Part model, mm, in its own coordinate system. A direction names the side the tool comes from. Round coordinates to 2 decimals unless told otherwise and drop trailing zeros. Loops run counter-clockwise (first coordinate to the right, second up) from the corner with the lowest first, then second, coordinate; pieces in that order, holes last.
1) Band-saw the part on C-C, the plane z = 8.25. Write the cut outline in (x, y).
2) 3-axis set-ups, long thin cutter, end or side, ignore diameter. For faces 1 (the flat face through (0, 8, 5)), 2 (the cylindrical face through (0, 2, 12)): which of +Z, -Z, +X, -X, +Y, -Y reach the whole face in a straight line?
3) Mould opens along Z. For faces 3 (the conical face through (-0.1, -5.2, 0.2)), 4 (the flat face through (0, 8, 13)), 5 (the flat face through (0, 3, 21)) say: +Z half, -Z half, draft (parallel to the pull), parting line (faces both ways), or undercut.
4) Band-saw the part on B-B, the plane z = 4.25. Write the cut outline in (x, y), then the cut area to 3 significant figures.
5) Probe line 1 (Z direction, x = 3, y = 7.5); line 2 (Y direction, x = 0, z = 8.5); line 3 (Y direction, x = 0, z = 15). List the from-to ranges inside material, lowest first.
6) Drop flat-ended pins along their axis: P1, Ø2, axis at y = -3, z = 3.5, coming from the -X side; P2, Ø8, axis at y = -4, z = 13.5, coming from the -X side; P3, Ø1.5, axis at y = -3, z = 12, coming from the +X side; P4, Ø2.5, axis at x = 2, z = 8, coming from the +Y side. Give the stop position or say it passes through.
Autodesk Inventor part; units mm, degrees
ref_plane "YZ Plane" through (0, 0, 0) normal (1, 0, 0) x (0, 1, 0)
ref_plane "XZ Plane" through (0, 0, 0) normal (0, 1, 0) x (-1, 0, 0)
ref_plane "XY Plane" through (0, 0, 0) normal (0, 0, 1) x (1, 0, 0)
sketch "Sketch2" plane through (0, 0, 0) normal (0, 0, 1) x (1, 0, 0)
  circle A0 centre (0, 0) radius 6
  circle A1 centre (0, 0) radius 2
  dimension "d0" = 12
  dimension "d1" = 4
extrude "Extrusion1" add sketch "Sketch2" along normal blind 21
sketch "Sketch3" plane through (0, 0, 21) normal (0, 0, 1) x (1, 0, 0)
  line L0 (0, 0) -> (0, 6) construction
  line L1 (6, 0) -> (6, 6)
  line L2 (-6, 6) -> (-6, 0)
  arc A0 (-6, 0) -> (6, 0) centre (0, 0) ccw
  arc A1 (6, 6) -> (-6, 6) centre (0, 6) ccw
  circle A2 centre (0, 0) radius 2
  circle A3 centre (0, 0) radius 6
  circle A4 centre (0, 0) radius 2
  circle A5 centre (0, 0) radius 6
  point P0 (0, 3)
  dimension "d4" = 6
  dimension "d5" = 6
extrude "Extrusion2" add sketch "Sketch3" against normal blind 8 contours A3 L2 A1 L1
sketch "Sketch4" plane through (0, 0, 0) normal (0, 0, -1) x (-1, 0, 0)
  arc A0 (6, 6) -> (-6, 6) centre (0, 6) ccw
  line L0 (-6, 6) -> (-6, 0)
  line L1 (6, 0) -> (6, 6)
  arc A1 (6, 0) -> (-6, 0) centre (0, 0) ccw
  circle A2 centre (0, 0) radius 2
extrude "Extrusion3" add sketch "Sketch4" against normal blind 5 contours L1 A1 L0 A0
sketch "Sketch5" plane through (0, 0, 13) normal (0, 0, -1) x (-1, 0, 0)
  arc A0 (6, 6) -> (-6, 6) centre (0, 6) ccw
  line L0 (-6, 6) -> (-6, 0)
  line L1 (6, 0) -> (6, 6)
  arc A1 (6, 0) -> (-6, 0) centre (0, 0) ccw
  line L2 (-6, 6) -> (6, 6)
  arc A2 (6, 0) -> (-6, 0) centre (0, 0) ccw
  point P0 (0, 6)
extrude "Extrusion4" add sketch "Sketch5" along normal blind 8.2 contours L1 A1 L2 | L2 A1 L0
chamfer "Chamfer1" distance 3 angle 45 1 edges at (-2, 0, 0)
chamfer "Chamfer2" distance 1 angle 45 4 edges at (-6, 3, 0) (0, 12, 0) (6, 3, 0) (0, -6, 0)
properties part number "picture-fixings-8mm"
Reported:
1. outline: (-6, 0) arc R6 ccw to (6, 0) - (6, 6) - (-6, 6) - close; hole circle Ø4 at (0, 0)
2. face 1: +X, -X, +Y
2. face 2: +Z, -Z
3. face 3: -Z half
3. face 4: undercut
3. face 5: +Z half
4. outline: (-6, 0) arc R6 ccw to (6, 0) - (6, 6) arc R6 ccw to (-6, 6) - close; hole circle Ø4 at (0, 0)
4. area: 173 mm2
5. line 1: z = 0 to 5, 13 to 21
5. line 2: y = -6 to -2, 2 to 6
5. line 3: y = -6 to -2, 2 to 12
6. P1: stops at x = -5.66
6. P2: stops at x = -6
6. P3: stops at x = 5.56
6. P4: stops at y = 6
